Check sheet for the modelled part. Datum: model origin and axes. Units: mm. Face numbers are marked on the shaded views. A direction names the side the tool comes from. Round coordinates to 2 decimals unless told otherwise and drop trailing zeros. Order: outer loops, then holes, each group sorted by start corner. A loop starts at its lowest first (then second) coordinate and runs counter-clockwise, first axis right, second up.
(1) Mould release check, pull along X, two halves, no side actions. Record for the marked faces 1, 2 and 3: released by +X, released by -X, zero draft, split by the parting line, or undercut.
(2) Sectioned sample at C-C, the plane y = 72. Enter the section's corners in (x, z).
(3) Sectioned sample at A-A, the plane z = 94. Enter the section's corners in (x, y).
(4) Tool access check on the marked faces 4 and 5. Record the directions out of +Z, -Z, +X, -X, +Y, -Y that give a thin tool (end or side, any length) a straight path to the whole face; none if there is none.
(5) Thickness scan on probe 1 along X at (y, z) = (606.5, 101); probe 2 along Y at (x, z) = (0, 6.75); probe 3 along Z at (x, y) = (-74, 364). Record the ranges inside material, lowest first.
(6) Sectioned sample at B-B, the plane y = 735.5. Enter the section's corners in (x, z), and give its area (3 significant figures).
(7) Sectioned sample at D-D, the plane x = 48.5. Enter the section's corners in (y, z).
(8) Depth check by flat-ended pin: pin 1 (12 mm diameter, centred on x = -98, y = -136, fed in from +Z); pin 2 (3 mm diameter, centred on x = -156.5, y = 800.5, fed in from +Z); pin 3 (6 mm diameter, centred on x = 0.5, z = 4.5, fed in from +Y). Enter the tip coordinate at first touch or a pass-through.
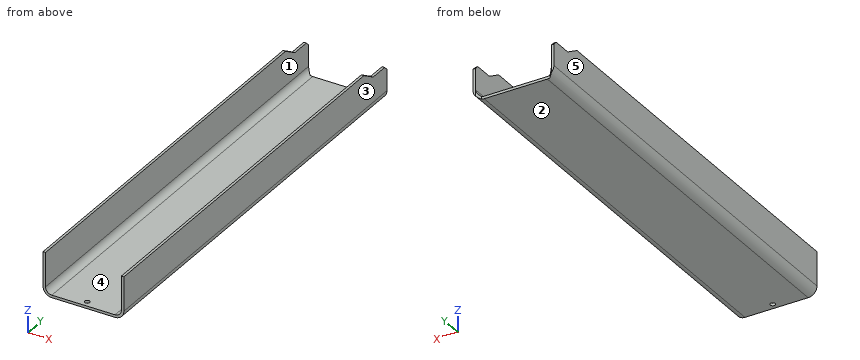
```python
from build123d import *

# Parameters (mm, degrees)
F1_DEPTH      = 854.5
F2_R          = 25
F3_R          = 35
F5_DEPTH      = 320.001
F7_D          = 20
F9_DEPTH      = 30
F9_DEPTH_BACK = 10


with BuildPart() as f1:
    # F0 (on Front) → F1 (new body, symmetric)
    with BuildSketch(Plane.XZ):
        Polygon((-150, 170), (-160, 170), (-160, 0), (160, 0), (160, 170), (150, 170), (150, 10), (-150, 10), align=None)
    extrude(amount=F1_DEPTH, both=True)

    # F2
    f2_edges = [f1.edges().sort_by_distance(p)[0] for p in [
        (-150, 0, 10),
        (150, 0, 10),
    ]]
    fillet(f2_edges, radius=F2_R)

    # F3
    f3_edges = [f1.edges().sort_by_distance(p)[0] for p in [
        (160, 0, 0),
        (-160, 0, 0),
    ]]
    fillet(f3_edges, radius=F3_R)

    # F4 (on face) → F5 (cut, through all)
    with BuildSketch(Plane.YZ.offset(160)):
        Polygon((854.5, 170), (704.5, 170), (764.5, 134), (839.5, 134), (854.5, 119), align=None)
    extrude(amount=-F5_DEPTH, mode=Mode.SUBTRACT)

    # F7 (through all)
    with Locations(Plane.XY.offset(10)):
        with Locations((0, -829.5)):
            Hole(F7_D / 2)

    # F8 (on face) → F9 (cut, two sides)
    with BuildSketch(Plane.XY.offset(10)) as f9_sk:
        Polygon((-150, 854.5), (-135, 839.5), (135, 839.5), (150, 854.5), align=None)
    extrude(amount=F9_DEPTH, mode=Mode.SUBTRACT)
    extrude(f9_sk.sketch, amount=-F9_DEPTH_BACK, mode=Mode.SUBTRACT)


solid = f1.part
```
Derived:
1. face 1: undercut
1. face 2: zero draft
1. face 3: released by +X
2. outline: (-160, 35) arc R35 ccw to (-125, 0) - (125, 0) arc R35 ccw to (160, 35) - (160, 170) - (150, 170) - (150, 35) arc R25 cw to (125, 10) - (-125, 10) arc R25 cw to (-150, 35) - (-150, 170) - (-160, 170) - close
3. outline: (-160, -854.5) - (-150, -854.5) - (-150, 854.5) - (-160, 854.5) - close; (150, -854.5) - (160, -854.5) - (160, 854.5) - (150, 854.5) - close
4. face 4: +Z, +Y, -Y
4. face 5: +Z, -Z, -X, +Y, -Y
5. probe 1: x = -160 to -150, 150 to 160
5. probe 2: y = -854.5 to -839.5, -819.5 to 839.5
5. probe 3: z = 0 to 10
6. outline: (-160, 35) arc R35 ccw to (-125, 0) - (125, 0) arc R35 ccw to (160, 35) - (160, 151.4) - (150, 151.4) - (150, 35) arc R25 cw to (125, 10) - (-125, 10) arc R25 cw to (-150, 35) - (-150, 151.4) - (-160, 151.4) - close
6. area: 5,770 mm2
7. outline: (-854.5, 0) - (839.5, 0) - (839.5, 10) - (-854.5, 10) - close
8. pin 1: stops at z = 10
8. pin 2: stops at z = 134
8. pin 3: stops at y = 839.5
